For this review, use the dimensioned drawing (mm, ordinates from the lowest corner) and the shaded views. A direction names the side the tool comes from. Coordinates: 2 decimals unless noted, no trailing zeros. Loops run counter-clockwise (first coordinate to the right, second up) from the corner with the lowest first, then second, coordinate; pieces in that order, holes last. Notation, with made-up numbers: M 75,-37.5 L 98,-37.5 A16 cw 98,-19.5 Z; hole C 48,85 d3. An arc over 180 degrees is marked long. One line per item, written item: value.
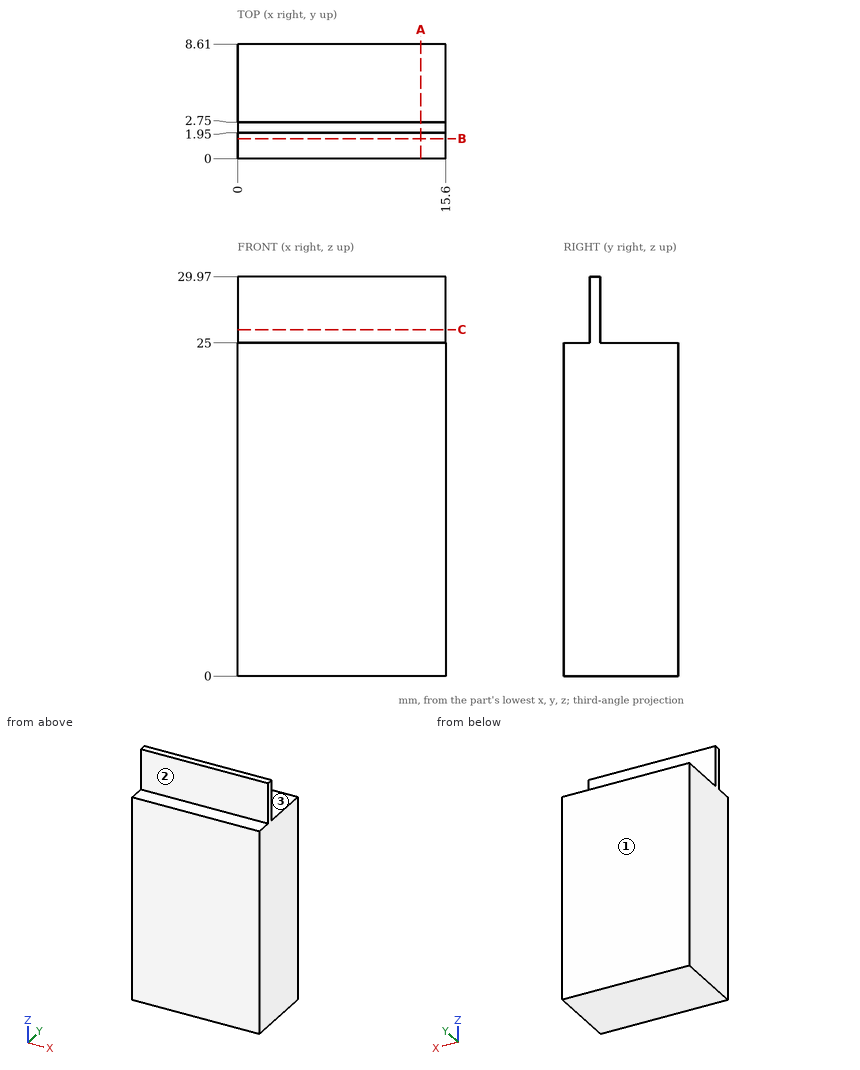
(1) Add section B-B on y = 1.5. State the section outline as (x, z) points.
Checks:
outline: M 0,0 L 15.6,0 L 15.6,25 L 0,25 Z
(2) Tool access review of the marked faces 1, 2 and 3: name each direction out of +Z, -Z, +X, -X, +Y, -Y from which nothing blocks a thin tool from reaching the whole face with its end or side.
Checks:
face 1: +Z, -Z, +X, -X, +Y
face 2: +Z, +X, -X, -Y
face 3: +Z, +X, -X, +Y
(3) Add section A-A on x = 13.75. State the section outline as (y, z) points.
Checks:
outline: M 0,0 L 8.61,0 L 8.61,25 L 2.75,25 L 2.75,29.97 L 1.95,29.97 L 1.95,25 L 0,25 Z
(4) Insertion check: pin 1 Ø3 at (x, y) = (11.5, 5) entering from +Z; pin 2 Ø4 at (x, z) = (5, 28.5) entering from -Y; pin 3 Ø4 at (x, z) = (4.5, 28.5) entering from +Y. Each pin has a flat end and moves straight along its axis. Give the tip position at first contact, or say it passes through.
Checks:
pin 1: z = 25
pin 2: y = 1.95
pin 3: y = 2.75
(5) Add section C-C on z = 26. State the section outline as (x, y) points.
Checks:
outline: M 0,1.95 L 15.6,1.95 L 15.6,2.75 L 0,2.75 Z
(6) To check wall thickness, follow L1, parallel to Z at x = 2, y = 1.5; L2, parallel to Y at x = 9, z = 27. State the ranges of each line that lie inside material, in increasing order. Write a range as [from, to].
Checks:
L1: [0, 25]
L2: [1.95, 2.75]
